Geometry check sheet. Reference: the model listing, model coordinates, mm. Round coordinates to 2 decimals unless told otherwise and drop trailing zeros. Write each loop counter-clockwise with the first axis right and the second up, starting at its lowest first coordinate (ties: lowest second). Pieces come first, ordered by that corner, then holes. Notation, with made-up numbers: (10.25, 31.5) - (21.25, 31.5) arc R24 ccw to (21.25, 52.5) - close; hole circle Ø6 at (34, -12). An arc over 180 degrees is marked (long way). One line per question, with ' | ' between items. Start each with the question number.
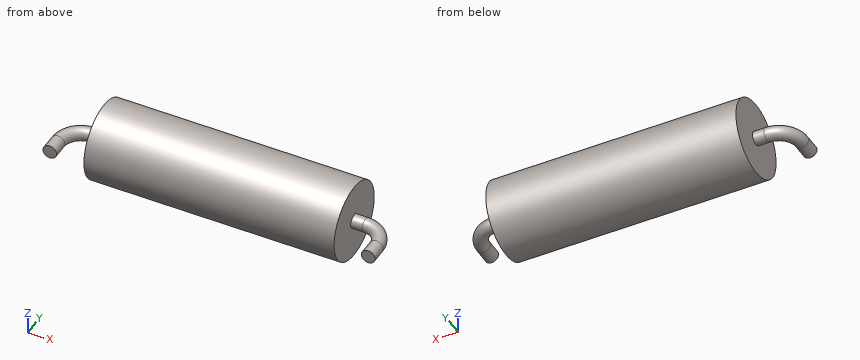
from build123d import *

# Parameters (mm, degrees)
SKETCH1_R                = 1.7
BOSS_EXTRUDE1_DEPTH      = 5.5
BOSS_EXTRUDE1_DEPTH_BACK = 5.5
SWEEP1_PROFILE_R         = 0.3


with BuildPart() as part:
    # Sketch1 → Boss-Extrude1 (new body, two sides)
    with BuildSketch(Plane(origin=(0, 0, 0), x_dir=(0, 0, -1), z_dir=(1, 0, 0))) as boss_extrude1_sk:
        Circle(SKETCH1_R)
    extrude(amount=BOSS_EXTRUDE1_DEPTH)
    extrude(boss_extrude1_sk.sketch, amount=-BOSS_EXTRUDE1_DEPTH_BACK)

    # Sweep1: sweep along a path in Sketch2
    with BuildLine(Plane.XY) as sweep1_path:
        Line((-5.5, 0), (-6, 0))
        ThreePointArc((-6, 0), (-6.707106781, -0.292893219), (-7, -1))
        Line((-7, -1), (-7, -1.7))
    # Sweep1 profile (on start of the path) → Sweep1 (sweep)
    with BuildSketch(Plane(origin=(-5.5, 0, 0), x_dir=(0, -1, 0), z_dir=(-1, 0, 0))):
        Circle(SWEEP1_PROFILE_R)
    sweep1 = sweep(path=sweep1_path.line)

    # Mirror1: Sweep1 across plane
    add(sweep1.mirror(Plane(origin=(0, 0, 0), x_dir=(0, 0, 1), z_dir=(1, 0, 0))))


solid = part.part
Q1. Section check B-B, the plane y = -1.3. Record the cut outline in (x, z).
Q2. Section check D-D, the plane y = 0.55. Record the cut outline in (x, z), then the cut area to 3 significant figures.
Q3. Section check C-C, the plane x = -2.75. Record the cut outline in (y, z), then the cut area to 3 significant figures.
Q4. Thickness scan on line 1 (X direction, y = 1.2, z = 0.35); line 2 (Z direction, x = -1.25, y = -1.45); line 3 (Y direction, x = 0.25, z = 1.05). Record the ranges inside material, lowest first.
Q5. Section check A-A, the plane z = 0. Record the cut outline in (x, y).
Q6. Go/stop test with flat-tipped pins: P1, Ø1, axis at x = -3.5, y = 1, coming from the -Z side; P2, Ø1.7, axis at y = 0.5, z = 0.5, coming from the -X side. Record where each tip stops, or that it passes through.
Result sheet:
1) outline: circle Ø0.6 at (-7, 0); (-5.5, -1.1) - (5.5, -1.1) - (5.5, 1.1) - (-5.5, 1.1) - close; circle Ø0.6 at (7, 0)
2) outline: (-5.5, -1.61) - (5.5, -1.61) - (5.5, 1.61) - (-5.5, 1.61) - close | area: 35.4 mm²
3) outline: circle Ø3.4 at (0, 0) | area: 9.08 mm²
4) line 1: -5.5 to 5.5 | line 2: -0.89 to 0.89 | line 3: -1.34 to 1.34
5) outline: (-7.3, -1.7) - (-6.7, -1.7) - (-6.7, -1) arc R0.7 cw to (-6, -0.3) - (-5.5, -0.3) - (-5.5, -1.7) - (5.5, -1.7) - (5.5, -0.3) - (6, -0.3) arc R0.7 cw to (6.7, -1) - (6.7, -1.7) - (7.3, -1.7) - (7.3, -1) arc R1.3 ccw to (6, 0.3) - (5.5, 0.3) - (5.5, 1.7) - (-5.5, 1.7) - (-5.5, 0.3) - (-6, 0.3) arc R1.3 ccw to (-7.3, -1) - close
6) P1: z = -1.62 | P2: x = -7.04
